Build history of the part. All positions in model axes, mm. Face numbers are marked on the shaded views. A direction names the side the tool comes from. Give positions to 0.01 mm unless a question says otherwise; leave off trailing zeros. Write each loop counter-clockwise with the first axis right and the second up, starting at its lowest first coordinate (ties: lowest second). Pieces come first, ordered by that corner, then holes. Notation, with made-up numbers: (48, 89) -> (57, 89) arc R28 ccw to (57, 123) -> close; hole circle Ø5 at (-9.5, 56). An arc over 180 degrees is marked (long way). Put each result on its own line as item: value.
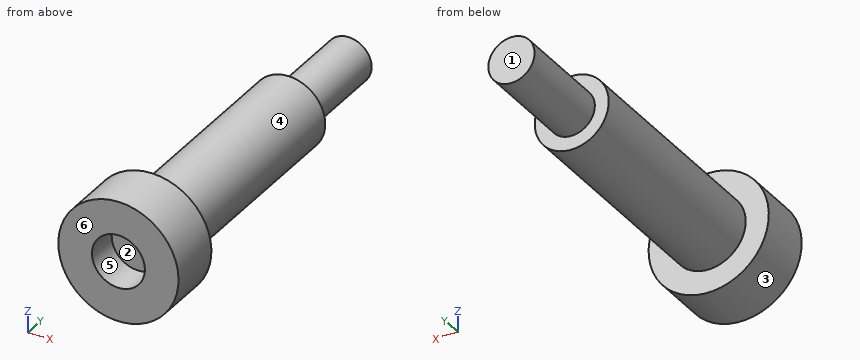
from build123d import *

# Parameters (mm, degrees)
ROSCA_START  = -3.175
CROQUIS1_R   = 2.5
ROSCA_DEPTH  = 11
HOMBRO_START = -28.175
CROQUIS2_R   = 4
HOMBRO_DEPTH = 25
CABEZA_START = -34.175
CROQUIS3_R   = 6.5
CABEZA_DEPTH = 6
ALLEN_START  = -34.175
CROQUIS4_R   = 2.86
ALLEN_DEPTH  = 3.6


with BuildPart() as part:
    # Croquis1 → Rosca (new body)
    with BuildSketch(Plane(origin=(0, 0, 0), x_dir=(1, 0, 0), z_dir=(0, 1, 0)).offset(ROSCA_START)):
        with Locations(Location((152.4, -336.55, 0), (0, 0, 270))):
            Circle(CROQUIS1_R)
    extrude(amount=ROSCA_DEPTH)

    # Croquis2 → Hombro (add)
    with BuildSketch(Plane(origin=(0, 0, 0), x_dir=(1, 0, 0), z_dir=(0, 1, 0)).offset(HOMBRO_START)):
        with Locations(Location((152.4, -336.55, 0), (0, 0, 270))):
            Circle(CROQUIS2_R)
    extrude(amount=HOMBRO_DEPTH)

    # Croquis3 → Cabeza (add)
    with BuildSketch(Plane(origin=(0, 0, 0), x_dir=(1, 0, 0), z_dir=(0, 1, 0)).offset(CABEZA_START)):
        with Locations(Location((152.4, -336.55, 0), (0, 0, 270))):
            Circle(CROQUIS3_R)
    extrude(amount=CABEZA_DEPTH)

    # Croquis4 → Allen (cut)
    with BuildSketch(Plane(origin=(0, 0, 0), x_dir=(1, 0, 0), z_dir=(0, 1, 0)).offset(ALLEN_START)):
        with Locations(Location((152.4, -336.55, 0), (0, 0, 270))):
            Circle(CROQUIS4_R)
    extrude(amount=ALLEN_DEPTH, mode=Mode.SUBTRACT)


solid = part.part
1) Pull direction X, two halves, no side cores. Call the marked faces 1, 2 and 3: released by +X, released by -X, zero draft, split by the parting line, or undercut.
Filled sheet:
face 1: zero draft
face 2: undercut
face 3: split by the parting line
2) Slice it at A-A (z = 336.55). Write the cut outline in (x, y) (3 decimals).
Filled sheet:
outline: (145.9, -34.175) -> (149.54, -34.175) -> (149.54, -30.575) -> (155.26, -30.575) -> (155.26, -34.175) -> (158.9, -34.175) -> (158.9, -28.175) -> (156.4, -28.175) -> (156.4, -3.175) -> (154.9, -3.175) -> (154.9, 7.825) -> (149.9, 7.825) -> (149.9, -3.175) -> (148.4, -3.175) -> (148.4, -28.175) -> (145.9, -28.175) -> close
3) Wall check: L1, parallel to X at y = -32.5, z = 336.55; L2, parallel to Y at x = 147.25, z = 337 (3 decimals); L3, parallel to Y at x = 154.75, z = 334.75 (3 decimals). Give the ranges that are in metal, low to high.
Filled sheet:
L1: 145.9 to 149.54, 155.26 to 158.9
L2: -34.175 to -28.175
L3: -34.175 to -3.175
4) Slice it at D-D (y = -19). Write the cut outline in (x, z), plus the area to 3 significant figures.
Filled sheet:
outline: circle Ø8 at (152.4, 336.55)
area: 50.3 mm2
5) Tool access for the marked faces 4, 5 and 6: list every direction of +Z, -Z, +X, -X, +Y, -Y with a clear straight run to the whole face (end or side of a thin tool).
Filled sheet:
face 4: +Y
face 5: -Y
face 6: +Z, -Z, +X, -X, -Y
6) Slice it at B-B (x = 152.4). Write the cut outline in (y, z) (3 decimals), plus the area to 3 significant figures.
Filled sheet:
outline: (-34.175, 330.05) -> (-28.175, 330.05) -> (-28.175, 332.55) -> (-3.175, 332.55) -> (-3.175, 334.05) -> (7.825, 334.05) -> (7.825, 339.05) -> (-3.175, 339.05) -> (-3.175, 340.55) -> (-28.175, 340.55) -> (-28.175, 343.05) -> (-34.175, 343.05) -> (-34.175, 339.41) -> (-30.575, 339.41) -> (-30.575, 333.69) -> (-34.175, 333.69) -> close
area: 312 mm2
7) Slice it at C-C (y = -29.5). Write the cut outline in (x, z).
Filled sheet:
outline: circle Ø13 at (152.4, 336.55)
8) Pin check, flat tips, straight feed: pin 1 (5 mm diameter, centred on x = 152.5, y = -22, fed in from -Z); pin 2 (6.5 mm diameter, centred on x = 150, z = 333.5, fed in from +Y) (3 decimals); pin 3 (1 mm diameter, centred on y = -4, z = 332, fed in from +X); pin 4 (1.5 mm diameter, centred on y = -27, z = 337.5, fed in from -X) (3 decimals). Stop position of each tip, or through.
Filled sheet:
pin 1: z = 332.55
pin 2: y = 7.825
pin 3: through
pin 4: x = 148.405
